Part model, mm, in its own coordinate system. Face numbers are marked on the shaded views. A direction names the side the tool comes from. Round coordinates to 2 decimals unless told otherwise and drop trailing zeros. Write each loop counter-clockwise with the first axis right and the second up, starting at its lowest first coordinate (ties: lowest second). Pieces come first, ordered by that corner, then holes. Notation, with made-up numbers: M 50,87.5 L 81,87.5 A32 ccw 81,113.5 Z; hole C -23.75,8 d5. An arc over 180 degrees is marked long. Answer as a JSON object with one key per item and string values. Group by question number.
1. Which spindle directions (+Z, -Z, +X, -X, +Y, -Y) get a long thin tool onto all of the face, cutting with end or side? Do the marked faces 1 and 2. Say none if no direction does.
2. Band-saw the part on C-C, the plane y = 1.75. Write the cut outline in (x, z).
3. Band-saw the part on B-B, the plane x = -1.25. Write the cut outline in (y, z), plus the area to 3 significant figures.
4. Band-saw the part on A-A, the plane y = 5.25. Count the separate pieces of the cut face and the enclosed holes in it, plus the area to 3 significant figures.
5. Drop flat-ended pins along their axis: pin 1 (2 mm diameter, centred on x = -10, y = 10.5, fed in from +Z); pin 2 (5 mm diameter, centred on x = -10.5, y = 10.5, fed in from +Z); pin 3 (1 mm diameter, centred on y = 2, z = 11.5, fed in from +X). Give the stop position or say it passes through.
6. Two-plate mould, pull along X, no slides. Class the marked faces 3, 4 and 5: +X half, -X half, draft (parallel to the pull), parting line (faces both ways), or undercut.
7. Drill centre lines: line 1 (X direction, y = 2, z = 0); line 2 (Y direction, x = 8, z = 2); line 3 (Z direction, x = -4.25, y = 6.25). Where is each one in solid material? Low to high. Write a range as from..to.
from build123d import *

# Parameters (mm, degrees)
SKETCH_1_R               = 15
SKETCH_1_R_2             = 2.5
EXTRUDE_1_DEPTH          = 3
SKETCH_2_R               = 1
EXTRUDE_2_DEPTH          = 10
PATTERN_CIRCULAR_1_COUNT = 15


with BuildPart() as part:
    # 草圖1 → 填料-伸長1 (new body)
    with BuildSketch(Plane(origin=(0, 0, 0), x_dir=(1, 0, 0), z_dir=(0, 1, 0))):
        with Locations(Location((0, 0, 0), (0, 0, 270))):
            Circle(SKETCH_1_R)
        with Locations(Location((0, 0, 0), (0, 0, 270))):
            Circle(SKETCH_1_R_2, mode=Mode.SUBTRACT)
    extrude(amount=EXTRUDE_1_DEPTH)

    # 草圖2 → 填料-伸長2 (add)
    with BuildSketch(Plane(origin=(0, 3, 0), x_dir=(1, 0, 0), z_dir=(0, 1, 0))):
        with Locations(Location((6.116820543, 10.901124091, 0), (0, 0, 270))):
            Circle(SKETCH_2_R)
    extrude_2 = extrude(amount=EXTRUDE_2_DEPTH)

    # 環狀複製排列1: 填料-伸長2 ×15 about axis
    pattern_circular_1_axis = Axis((0, 0, 0), (0, 1, 0))
    for i in range(1, PATTERN_CIRCULAR_1_COUNT):
        add(extrude_2.rotate(pattern_circular_1_axis, i * 360 / PATTERN_CIRCULAR_1_COUNT))


solid = part.part
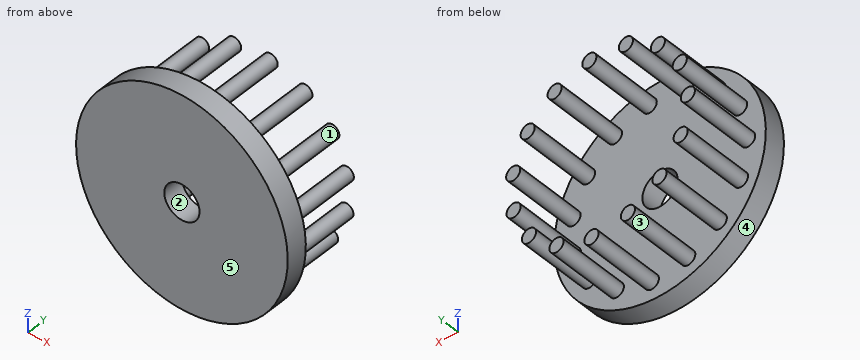
Worked answers:
{
 "1": {"face 1": "+Y", "face 2": "+Y, -Y"},
 "2": {"outline": "C 0,0 d30; hole C 0,0 d5"},
 "3": {"outline": "M 0,-14.95 L 3,-14.95 L 3,-2.17 L 0,-2.17 Z; M 0,2.17 L 3,2.17 L 3,14.95 L 0,14.95 Z", "area": "76.7 mm^2"},
 "4": {"separate pieces": "15", "enclosed holes": "0", "area": "47.1 mm^2"},
 "5": {"pin 1": "stops at z = 10.05", "pin 2": "stops at z = 10.39", "pin 3": "stops at x = 10.2"},
 "6": {"face 3": "undercut", "face 4": "parting line", "face 5": "draft"},
 "7": {"line 1": "x = -15..-2.5, 2.5..15", "line 2": "y = 0..3", "line 3": "z = -12.81..-10.87, 11.09..12.78"}
}
